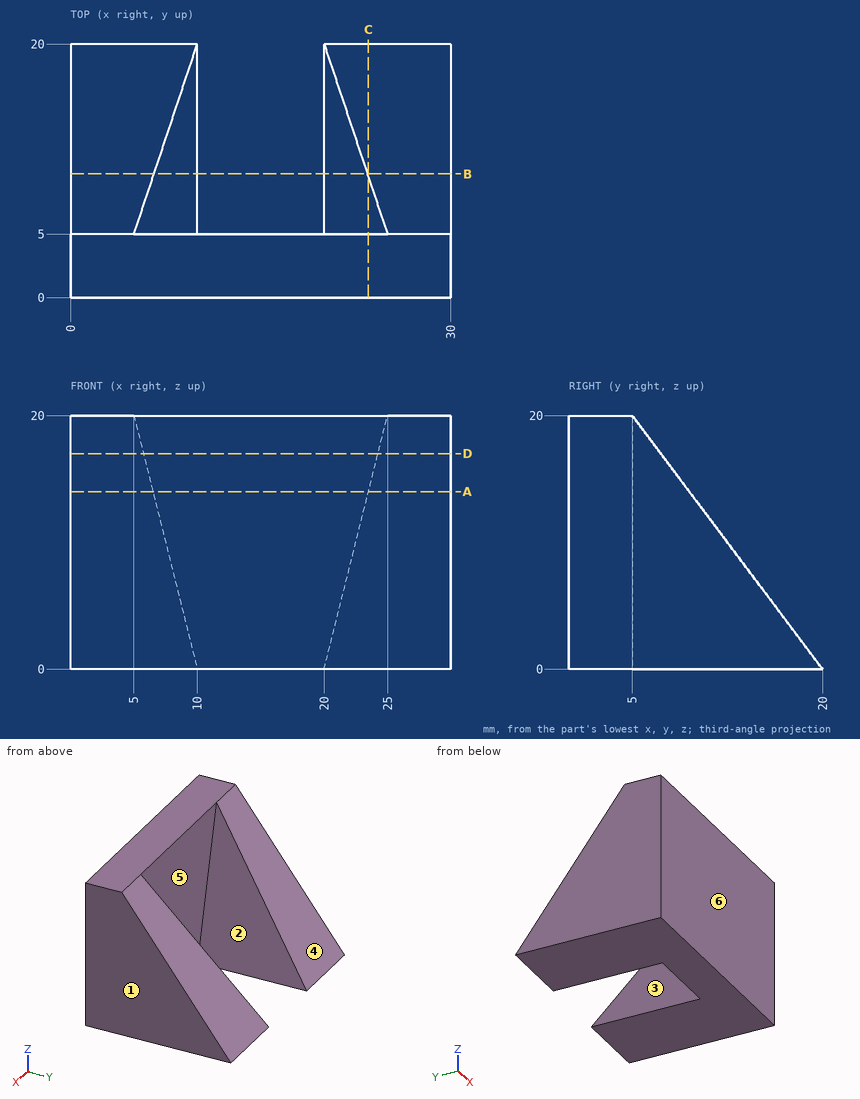
For this review, use the dimensioned drawing (mm, ordinates from the lowest corner) and the shaded views. A direction names the side the tool comes from. Give positions to 0.01 mm unless a question says otherwise; leave off trailing zeros. Loops run counter-clockwise (first coordinate to the right, second up) from the corner with the lowest first, then second, coordinate; pieces in that order, holes last. Notation, with made-up numbers: (-24.5, 13.5) - (1.5, 13.5) arc R21 cw to (1.5, 36.5) - close; hole circle Ø10 at (77.25, -15.75). An arc over 180 degrees is marked (long way). Write each question's results on one line, items separated by ' | '.
(1) Draft analysis for pull direction X (two halves, no side actions). For the marked faces 1, 2, 3 and 4, state which applies: +X half, -X half, draft (parallel to the pull), parting line (faces both ways), or undercut.
Conclusion:
face 1: +X half | face 2: undercut | face 3: undercut | face 4: draft
(2) For the marked faces 5 and 6, list the 3-axis set-ups (+Z, -Z, +X, -X, +Y, -Y) from which the entire face can be reached by the end or side of a thin tool; tool diameter is ignored.
Conclusion:
face 5: +Z, +Y | face 6: +Z, -Z, +X, -X, -Y
(3) Take a section at C-C (x = 23.5). Give the boundary of the cut face in (y, z).
Conclusion:
outline: (0, 0) - (20, 0) - (9.5, 14) - (5, 14) - (5, 20) - (0, 20) - close
(4) For line 1 along Y through (x, z) = (14, 6.75); line 2 along X through (y, z) = (14.25, 7.5) (3 decimals); line 3 along X through (y, z) = (7.25, 14), list the stretches that pass through material, from the lowest coordinate up.
Conclusion:
line 1: 0 to 5 | line 2: 0 to 8.125, 21.875 to 30 | line 3: 0 to 6.5, 23.5 to 30
(5) Take a section at A-A (z = 14). Give the boundary of the cut face in (x, y), then the cut area to 4 significant figures.
Conclusion:
outline: (0, 0) - (30, 0) - (30, 9.5) - (23.5, 9.5) - (23.5, 5) - (6.5, 5) - (6.5, 9.5) - (0, 9.5) - close | area: 208.5 mm^2
(6) Take a section at B-B (y = 9.75). Give the boundary of the cut face in (x, z), then the cut area to 3 significant figures.
Conclusion:
outline: (0, 0) - (10, 0) - (6.58, 13.67) - (0, 13.67) - close; (20, 0) - (30, 0) - (30, 13.67) - (23.42, 13.67) - close | area: 227 mm^2
(7) For pin 1 Ø8 at (x, z) = (16, 8.5) entering from +Y; pin 2 Ø2 at (x, z) = (3.5, 12.5) entering from +Y (3 decimals); pin 3 Ø6 at (x, y) = (5.5, 11) entering from +Z, all flat-tipped, find the tip position at first contact; note any pin that passes through.
Conclusion:
pin 1: y = 5 | pin 2: y = 11.375 | pin 3: z = 16
(8) Take a section at D-D (z = 17). Give the boundary of the cut face in (x, y).
Conclusion:
outline: (0, 0) - (30, 0) - (30, 7.25) - (24.25, 7.25) - (24.25, 5) - (5.75, 5) - (5.75, 7.25) - (0, 7.25) - close
